CAD build for the part. Positions are in the model's coordinates, mm. A direction names the side the tool comes from. Give positions to 0.01 mm unless a question says otherwise; leave off trailing zeros. Loops run counter-clockwise (first coordinate to the right, second up) from the corner with the lowest first, then second, coordinate; pieces in that order, holes last.
Item 1: Saw through at D-D on z = -29. Give the cut face in (x, y).
Item 2: Saw through at A-A on x = -18. Give the cut face in (y, z), plus the area to 3 significant figures.
Item 3: Mould opens along X. For faces 3 (the cylindrical face through (5.326, 98.6, -7.729)), 4 (the flat face through (-31, 0, -4)), 5 (the flat face through (-24.419, 99, -11)) say: released by +X, released by -X, zero draft, split by the parting line, or undercut.
Item 4: Saw through at B-B on z = -17.5. Give the cut face in (x, y).
Item 5: Saw through at C-C on x = -33. Give the cut face in (y, z), plus the area to 3 significant figures.
Item 6: Drop flat-ended pins along their axis: P1, Ø6.5, axis at y = 135, z = -20.5, coming from the +X side; P2, Ø8, axis at x = -40, z = 1.5, coming from the -Y side; P3, Ø0.8, axis at y = 56.5, z = 6, coming from the -X side; P4, Ø2, axis at x = -26.5, y = 28.5, coming from the +Z side. Give the stop position or say it passes through.
Item 7: Which spindle directions (+Z, -Z, +X, -X, +Y, -Y) get a long thin tool onto all of the face, cutting with end or side? Do faces 1 (the flat face through (-31, 200, -4)), 2 (the cylindrical face through (-2.424, 98.6, -4.301)). Say none if no direction does.
Item 8: Probe probe 1 along X at (y, z) = (176.5, -3); probe 2 along X at (y, z) = (169.5, 1.5); probe 3 along Z at (x, y) = (-23, 34). List the from-to ranges inside material, lowest first.
from build123d import *

# Parameters (mm, degrees)
SKETCH1_R           = 30
BOSS_EXTRUDE2_DEPTH = 200
FILLET1_R           = 0.5


with BuildPart() as part:
    # Sketch1 → Boss-Extrude2 (new body)
    # profile 1 of 2: a face of its own
    with BuildSketch(Plane(origin=(0, 0, 0), x_dir=(1, 0, 0), z_dir=(0, 1, 0))):
        with Locations(Location((-24.418699654, 3.823974383, 0), (0, 0, 270))):
            Circle(SKETCH1_R)
        with BuildLine():
            Line((-26.418699654, -18.176025617), (-26.418699654, -4.176025617))
            Line((-26.418699654, -4.176025617), (-26.418699654, -3.176025617))
            Line((-26.418699654, -3.176025617), (-26.418699654, 10.823974383))
            Line((-26.418699654, 10.823974383), (-25.418699654, 10.823974383))
            Line((-25.418699654, 10.823974383), (-25.418699654, 7.323974383))
            Line((-25.418699654, 7.323974383), (-24.418699654, 7.323974383))
            Line((-24.418699654, 7.323974383), (-24.418699654, 10.823974383))
            Line((-24.418699654, 10.823974383), (-24.418699654, 11.823974383))
            Line((-24.418699654, 11.823974383), (-24.418699654, 15.323974383))
            Line((-24.418699654, 15.323974383), (-25.418699654, 15.323974383))
            Line((-25.418699654, 15.323974383), (-25.418699654, 11.823974383))
            Line((-25.418699654, 11.823974383), (-26.418699654, 11.823974383))
            Line((-26.418699654, 11.823974383), (-26.418699654, 25.823974383))
            Line((-26.418699654, 25.823974383), (-25.418699654, 25.823974383))
            Line((-25.418699654, 25.823974383), (-25.418699654, 22.323974383))
            Line((-25.418699654, 22.323974383), (-24.418699654, 22.323974383))
            Line((-24.418699654, 22.323974383), (-24.418699654, 25.823974383))
            ThreePointArc((-24.418699654, 25.823974383), (-2.418699654, 3.823974383), (-24.418699654, -18.176025617))
            Line((-24.418699654, -18.176025617), (-24.418699654, -14.676025617))
            Line((-24.418699654, -14.676025617), (-25.418699654, -14.676025617))
            Line((-25.418699654, -14.676025617), (-25.418699654, -18.176025617))
            Line((-25.418699654, -18.176025617), (-26.418699654, -18.176025617))
        make_face(mode=Mode.SUBTRACT)
    # profile 2 of 2: a face of its own
    with BuildSketch(Plane(origin=(0, 0, 0), x_dir=(1, 0, 0), z_dir=(0, 1, 0))):
        Polygon((-26.418699654, -3.176025617), (-26.418699654, -4.176025617), (-25.418699654, -4.176025617), (-25.418699654, -7.676025617), (-24.418699654, -7.676025617), (-24.418699654, -4.176025617), (-24.418699654, -3.176025617), (-24.418699654, 0.323974383), (-25.418699654, 0.323974383), (-25.418699654, -3.176025617), align=None)
    extrude(amount=BOSS_EXTRUDE2_DEPTH)

    # Fillet1
    fillet1_edges = [part.edges().sort_by_distance(p)[0] for p in [
        (-24.418699654, 100, -25.823974383),
        (-25.418699654, 100, 3.176025617),
        (-25.418699654, 100, -0.323974383),
        (-25.418699654, 100, -15.323974383),
        (-25.418699654, 100, -11.823974383),
        (-25.418699654, 100, -25.823974383),
        (-25.418699654, 100, -22.323974383),
        (-25.418699654, 100, -7.323974383),
        (-25.418699654, 100, -10.823974383),
        (-25.418699654, 100, 4.176025617),
        (-24.418699654, 100, -0.323974383),
        (-24.418699654, 100, -15.323974383),
        (-26.418699654, 100, -11.823974383),
        (-26.418699654, 100, 3.176025617),
        (-26.418699654, 100, -25.823974383),
        (-24.418699654, 100, -22.323974383),
        (-24.418699654, 100, -7.323974383),
        (-26.418699654, 100, -10.823974383),
        (-26.418699654, 100, 4.176025617),
        (-24.418699654, 100, 7.676025617),
        (-25.418699654, 100, 7.676025617),
        (-25.418699654, 100, 14.676025617),
        (-24.418699654, 100, 14.676025617),
        (-24.418699654, 100, 18.176025617),
        (-26.418699654, 100, 18.176025617),
        (-25.418699654, 100, 18.176025617),
    ]]
    fillet(fillet1_edges, radius=FILLET1_R - 0.0001)  # a hair under: the kernel refuses the full size


solid = part.part
Results below:
1. outline: (-40.73, 0) - (-8.1, 0) - (-8.1, 200) - (-40.73, 200) - close
2. outline: (0, -33.13) - (200, -33.13) - (200, -24.87) - (0, -24.87) - close; (0, 17.22) - (200, 17.22) - (200, 25.48) - (0, 25.48) - close
2. area: 3,300 mm2
3. face 3: split by the parting line
3. face 4: zero draft
3. face 5: undercut
4. outline: (-51.12, 0) - (-26.42, 0) - (-26.42, 200) - (-51.12, 200) - close; (-7.19, 0) - (2.28, 0) - (2.28, 200) - (-7.19, 200) - close
5. outline: (0, -32.57) - (200, -32.57) - (200, 24.92) - (0, 24.92) - close
5. area: 11,500 mm2
6. P1: stops at x = 2.41
6. P2: stops at y = 0
6. P3: stops at x = -52.9
6. P4: stops at z = 26.16
7. face 1: +Z, -Z, +X, -X, +Y
7. face 2: +Y, -Y
8. probe 1: x = -54.41 to -26.42, -2.43 to 5.57
8. probe 2: x = -53.94 to -26.42, -25.42 to -24.42, -3.07 to 5.11
8. probe 3: z = -33.79 to -25.78, 18.13 to 26.14
